Can you work these out from the drawing? Everything is in mm from the part's minimum corner. Give positions to 0.01 mm unless a question says otherwise; leave off trailing zeros. Order: outer loops, then holes, each group sorted by start corner. A loop starts at its lowest first (then second) coordinate and runs counter-clockwise, first axis right, second up. Notation, with made-up numbers: (-17, 9) - (9, 9) arc R11 ccw to (9, 29) - close; hole circle Ø5 at (6.25, -20.5). An arc over 180 degrees is marked (long way). Answer as a JSON object with one key per item and string values.
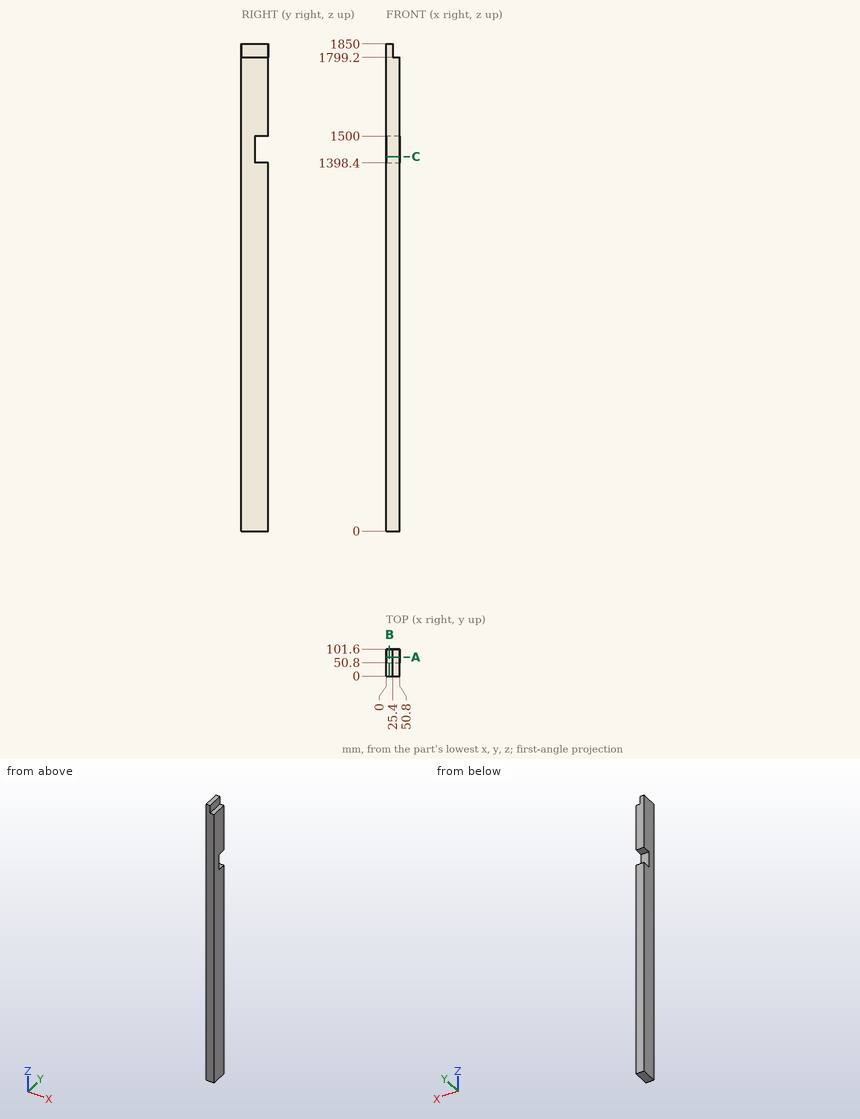
Q1. If we section it at B-B, the plane x = 12: Please give me the cut outline in (y, z), then the cut area to 3 significant figures.
Recorded:
{"outline": "(0, 0) - (101.6, 0) - (101.6, 1398.4) - (50.8, 1398.4) - (50.8, 1500) - (101.6, 1500) - (101.6, 1850) - (0, 1850) - close", "area": "183,000 mm^2"}
Q2. If we section it at A-A, the plane y = 71.5: Please give me the cut outline in (x, z), then the cut area to 3 significant figures.
Recorded:
{"outline": "(0, 0) - (50.8, 0) - (50.8, 1398.4) - (0, 1398.4) - close; (0, 1500) - (50.8, 1500) - (50.8, 1799.2) - (25.4, 1799.2) - (25.4, 1850) - (0, 1850) - close", "area": "87,500 mm^2"}
Q3. I need wall thicknesses on L1, parallel to Z at x = 34, y = 77; L2, parallel to Z at x = 13.5, y = 71; L3, parallel to Y at x = 41.5, z = 1448. Which ranges of each line are inside material? Lowest first, please.
Recorded:
{"L1": "z = 0 to 1398.4, 1500 to 1799.2", "L2": "z = 0 to 1398.4, 1500 to 1850", "L3": "y = 0 to 50.8"}
Q4. I'm going to push flat-ended pins straight in: pin 1 Ø6 at (x, z) = (8.5, 747.5) entering from -Y; pin 2 Ø2 at (x, z) = (23.5, 1458.5) entering from +Y. Where does each tip first touch, or does it pass through?
Recorded:
{"pin 1": "stops at y = 0", "pin 2": "stops at y = 50.8"}
Q5. If we section it at C-C, the plane z = 1422: Please give me the cut outline in (x, y).
Recorded:
{"outline": "(0, 0) - (50.8, 0) - (50.8, 50.8) - (0, 50.8) - close"}
